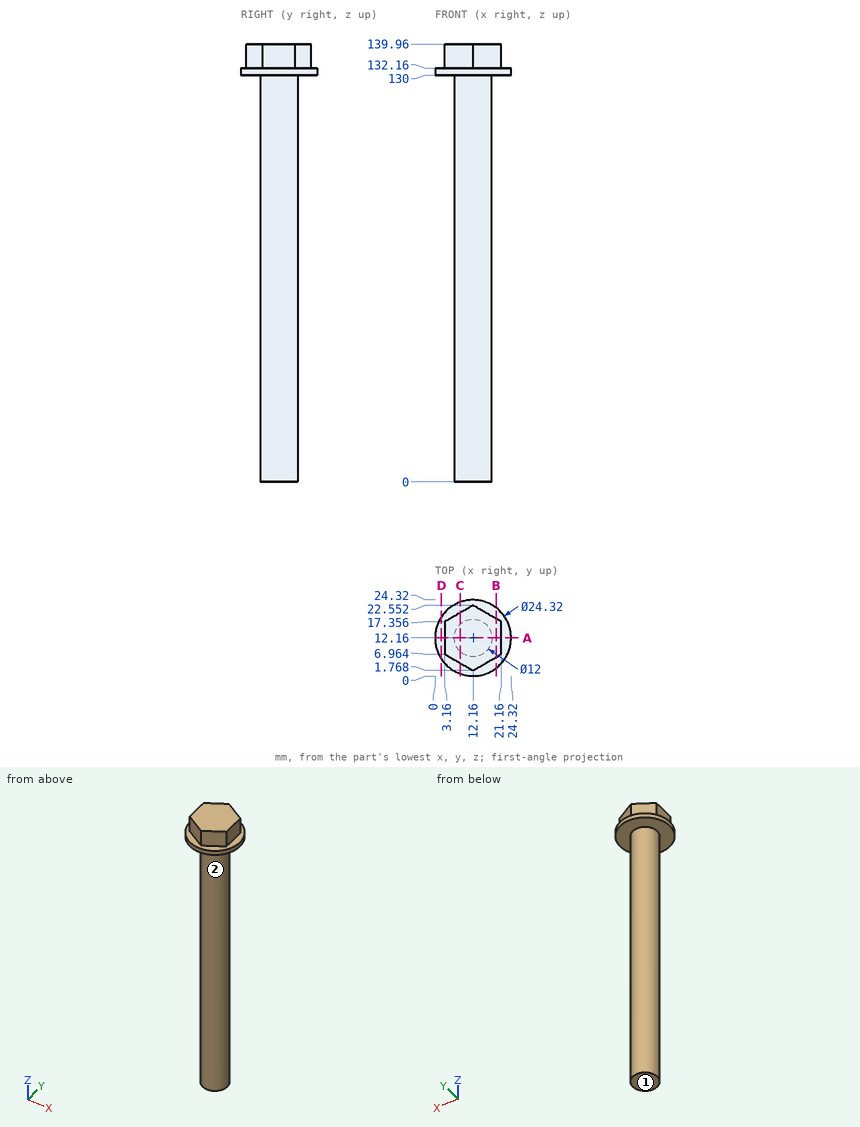
Can you work these out from the drawing? Everything is in mm from the part's minimum corner. A direction names the side the tool comes from. Round coordinates to 2 decimals unless told otherwise and drop trailing zeros. Loops run counter-clockwise (first coordinate to the right, second up) from the corner with the lowest first, then second, coordinate; pieces in that order, holes last. Notation, with made-up numbers: M 16.25,25 L 45.25,25 A22 ccw 45.25,57 Z; hole C -10.5,-35.5 d3. An arc over 180 degrees is marked long. Answer in a Markdown table with one row per item.
1. If we section it at B-B, the plane x = 19.5: Please give me the cut outline in (y, z) (1 decimal).
Established:
| item | result |
|---|---|
| outline | M 2.5,130 L 21.9,130 L 21.9,132.2 L 18.3,132.2 L 18.3,140 L 6,140 L 6,132.2 L 2.5,132.2 Z |
2. On a 3-axis mill with a long thin cutter (end or side, diameter ignored), from which of +Z, -Z, +X, -X, +Y, -Y can I reach the whole of each face in a straight line? I mean the marked faces 1 and 2. Say none if no direction works.
Established:
| item | result |
|---|---|
| face 1 | -Z, +X, -X, +Y, -Y |
| face 2 | -Z |
3. If we section it at C-C, the plane x = 8: Please give me the cut outline in (y, z).
Established:
| item | result |
|---|---|
| outline | M 0.73,130 L 7.84,130 L 7.84,0 L 16.48,0 L 16.48,130 L 23.59,130 L 23.59,132.16 L 20.15,132.16 L 20.15,139.96 L 4.17,139.96 L 4.17,132.16 L 0.73,132.16 Z |
4. If we section it at A-A, the plane y = 12.16: Please give me the cut outline in (x, z), plus the area to 3 significant figures.
Established:
| item | result |
|---|---|
| outline | M 0,130 L 6.16,130 L 6.16,0 L 18.16,0 L 18.16,130 L 24.32,130 L 24.32,132.16 L 21.16,132.16 L 21.16,139.96 L 3.16,139.96 L 3.16,132.16 L 0,132.16 Z |
| area | 1,750 mm² |
5. Please list where these lines run through material, in increasing order: line 1 (Z direction, x = 23.25, y = 13.5); line 2 (Z direction, x = 4.75, y = 12.25); line 3 (X direction, y = 12.25, z = 121). Write a range as from..to.
Established:
| item | result |
|---|---|
| line 1 | 130..132.16 |
| line 2 | 130..139.96 |
| line 3 | 6.16..18.16 |
6. I'm going to push flat-ended pins straight in: pin 1 Ø2.5 at (y, z) = (14.5, 135) entering from +X; pin 2 Ø1.5 at (y, z) = (14, 17.5) entering from +X; pin 3 Ø6 at (x, y) = (21.5, 20) entering from -Z. Where does each tip first touch, or does it pass through?
Established:
| item | result |
|---|---|
| pin 1 | x = 21.16 |
| pin 2 | x = 18.06 |
| pin 3 | z = 130 |
7. If we section it at D-D, the plane x = 2: Please give me the cut outline in (y, z).
Established:
| item | result |
|---|---|
| outline | M 5.48,130 L 18.84,130 L 18.84,132.16 L 5.48,132.16 Z |
